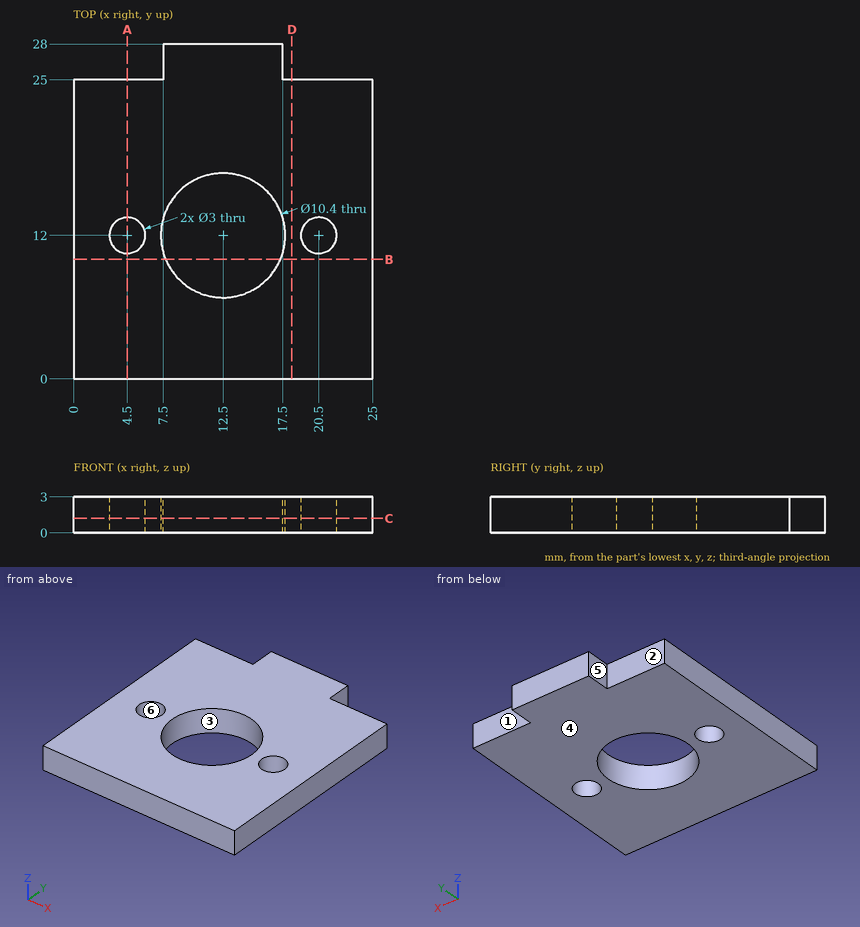
Check sheet for the drawn part. Datum: minimum x, y, z corner. Units: mm. A direction names the side the tool comes from. Coordinates: 2 decimals unless noted, no trailing zeros. Write each loop counter-clockwise with the first axis right and the second up, starting at its lowest first coordinate (ties: lowest second). Pieces come first, ordered by that corner, then holes. Notation, with made-up numbers: M 3,78.25 L 22,78.25 A18 ccw 22,113.25 Z; hole C 13,34.25 d3. An arc over 180 degrees is marked long. One line per item, written item: value.
Item 1: Section check A-A, the plane x = 4.5. Record the boundary of the cut face in (y, z), plus the area to 3 significant figures.
Check sheet entries:
outline: M 0,0 L 10.5,0 L 10.5,3 L 0,3 Z; M 13.5,0 L 25,0 L 25,3 L 13.5,3 Z
area: 66.0 mm^2
Item 2: Mould release check, pull along X, two halves, no side actions. Record for the marked faces 4, 5 and 6: pulls with the +X half, pulls with the -X half, needs draft (parallel to the pull), parting line crosses it, or undercut.
Check sheet entries:
face 4: needs draft
face 5: pulls with the -X half
face 6: undercut
Item 3: Section check C-C, the plane z = 1.2. Record the boundary of the cut face in (x, y), plus the area to 3 significant figures.
Check sheet entries:
outline: M 0,0 L 25,0 L 25,25 L 17.5,25 L 17.5,28 L 7.5,28 L 7.5,25 L 0,25 Z; hole C 4.5,12 d3; hole C 12.5,12 d10.4; hole C 20.5,12 d3
area: 556 mm^2
Item 4: Access from +Z, -Z, +X, -X, +Y, -Y to the whole of each face (thin tool, end or side, straight path). Record for the marked faces 1, 2 and 3.
Check sheet entries:
face 1: +Z, -Z, +X, +Y
face 2: +Z, -Z, -X, +Y
face 3: +Z, -Z
Item 5: Section check B-B, the plane y = 10. Record the boundary of the cut face in (x, z).
Check sheet entries:
outline: M 0,0 L 7.7,0 L 7.7,3 L 0,3 Z; M 17.3,0 L 25,0 L 25,3 L 17.3,3 Z
Item 6: Scan lines: line 1 along Y through (x, z) = (12.5, 1.1); line 2 along Y through (x, z) = (20.5, 0.25); line 3 along X through (y, z) = (10, 2.15). Record each from-to range of solid material in increasing order.
Check sheet entries:
line 1: y = 0 to 6.8, 17.2 to 28
line 2: y = 0 to 10.5, 13.5 to 25
line 3: x = 0 to 7.7, 17.3 to 25
Item 7: Section check D-D, the plane x = 18.25. Record the boundary of the cut face in (y, z), plus the area to 3 significant figures.
Check sheet entries:
outline: M 0,0 L 25,0 L 25,3 L 0,3 Z
area: 75.0 mm^2
Item 8: Gauge pin test, flat ends, axial feed: pin 1 Ø1.5 at (y, z) = (27, 1) entering from -X; pin 2 Ø1.5 at (x, z) = (2.5, 1.5) entering from +Y; pin 3 Ø0.9 at (y, z) = (26.5, 1) entering from +X. Record the tip position at first contact, or that the pin passes through.
Check sheet entries:
pin 1: stops at x = 7.5
pin 2: stops at y = 25
pin 3: stops at x = 17.5
